Part print with two shaded views. Sizes in mm from the minimum x, y, z corner. A direction names the side the tool comes from. Round coordinates to 2 decimals unless told otherwise and drop trailing zeros. Write each loop counter-clockwise with the first axis right and the second up, starting at its lowest first coordinate (ties: lowest second). Pieces come first, ordered by that corner, then holes. Notation, with made-up numbers: M -38,78.25 L -28,78.25 A24 ccw -28,102.25 Z; hole C -15.5,-19.5 d2. An arc over 180 degrees is marked long. Use one line per item in the form item = value. Start each with the question number.
Item 1: Probe L1, parallel to X at y = 18.5, z = 18.25 (1 decimal); L2, parallel to Z at x = 46.5, y = 14; L3, parallel to X at y = 13.75, z = 20.5 (1 decimal). List the from-to ranges inside material, lowest first.
Item 2: Flat gauge pins, fed straight in: pin 1 Ø3 at (x, y) = (15.5, 15.5) entering from -Z; pin 2 Ø4 at (x, y) = (9, 11) entering from -Z; pin 3 Ø5 at (x, y) = (22, 14) entering from +Z (1 decimal). Where does each tip first touch, or does it go through?
Item 3: Which spindle directions (+Z, -Z, +X, -X, +Y, -Y) get a long thin tool onto all of the face, cutting with end or side? Do the marked faces 1 and 2. Say none if no direction does.
Item 4: Cut at B-B, the plane x = 43.5. Give the cut face in (y, z).
Item 5: Mould opens along Z. For the marked faces 3, 4, 5 and 6 say: +Z half, -Z half, draft (parallel to the pull), parting line (faces both ways), or undercut.
Item 6: Cut at D-D, the plane x = 33.5. Give the cut face in (y, z), then the cut area to 3 significant figures.
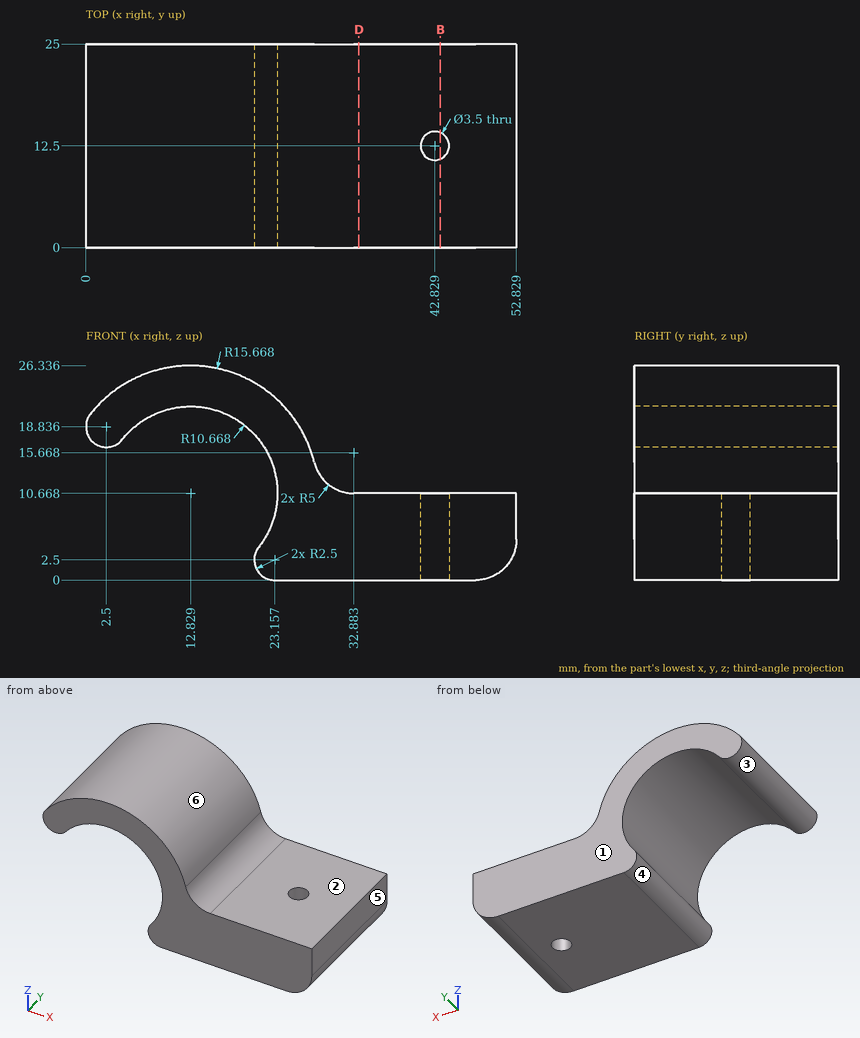
Model answer:
q1.L1 = 0.1 to 5.3, 20.3 to 26.5
q1.L2 = 0 to 10.67
q1.L3 = 0.6 to 8.7, 17 to 25
q2.pin_1 = 20.49
q2.pin_2 = 19.6
q2.pin_3 = 24.8
q3.face_1 = +Z, -Z, +X, -X, +Y
q3.face_2 = +Z, +X, +Y, -Y
q4.outline = M 0,0 L 10.88,0 L 10.88,10.67 L 0,10.67 Z; M 14.12,0 L 25,0 L 25,10.67 L 14.12,10.67 Z
q5.face_3 = parting line
q5.face_4 = undercut
q5.face_5 = draft
q5.face_6 = +Z half
q6.outline = M 0,0 L 25,0 L 25,10.67 L 0,10.67 Z
q6.area = 267 mm²
